Source: CAD feature listing. Evaluate the final solid. Frame: model axes, mm. Give positions to 0.01 mm unless a question says otherwise; leave off trailing zeros. Order: outer loops, then holes, each group sorted by start corner. A loop starts at its lowest first (then second) coordinate and runs counter-clockwise, first axis right, second up. Notation, with made-up numbers: M 87,49.25 L 146,49.25 A17 ccw 146,55.25 Z; hole C 43.5,-6.5 d7. An arc over 180 degrees is marked long. Answer as a JSON object with one key per item and string values. Group by question number.
1. Pin query (flat end, axial travel): P1, Ø1.6, axis at x = 46.99, y = 22.86, coming from the +Z side. Return the tip coordinate at first contact, or that it passes through.
2. Material intervals for L1, parallel to Y at x = 43.18, z = 0.45; L2, parallel to Y at x = 72.39, z = 1.2; L3, parallel to X at y = 10, z = 0.2, sorted ascending. Write a range as [from, to].
3. Pull-direction query (X, two-part tool) for faces 1 (the cylindrical face through (18.45, 2.98, 0.79)), 2 (the flat face through (5.08, 15, 1)), 3 (the cylindrical face through (94.47, 4.54, 0.79)), 4 (the flat face through (50, 0, 1)); classes: +X half, -X half, draft (parallel to the pull), parting line (faces both ways), or undercut.
4. Section query B-B (z = 0.3). Count the separate pieces of the cut face and the enclosed holes in it, plus the area to 3 significant figures.
5. Section query A-A (x = 72.39). Output: boundary loops of the cut face in (y, z).
Autodesk Inventor part; units mm, degrees
ref_plane "YZ Plane" through (0, 0, 0) normal (1, 0, 0) x (0, 1, 0)
ref_plane "XZ Plane" through (0, 0, 0) normal (0, 1, 0) x (-1, 0, 0)
ref_plane "XY Plane" through (0, 0, 0) normal (0, 0, 1) x (1, 0, 0)
sketch "Эскиз1" plane through (0, 0, 0) normal (0, 0, 1) x (1, 0, 0)
  line L0 (5.08, 0) -> (97.079, 0)
  line L1 (97.079, 0) -> (97.079, 30.47)
  line L2 (97.079, 30.47) -> (5.08, 30.47)
  line L3 (5.08, 30.47) -> (5.08, 0)
  circle A0 centre (46.99, 22.86) radius 0.6
  circle A1 centre (46.99, 20.32) radius 0.6
  circle A2 centre (46.99, 17.78) radius 0.6
  circle A3 centre (46.99, 15.24) radius 0.6
  circle A4 centre (46.99, 12.7) radius 0.6
  circle A5 centre (46.99, 10.16) radius 0.6
  circle A6 centre (46.99, 7.62) radius 0.6
  circle A7 centre (46.99, 5.08) radius 0.6
  circle A8 centre (54.61, 5.08) radius 0.6
  circle A9 centre (54.61, 7.62) radius 0.6
  circle A10 centre (54.61, 10.16) radius 0.6
  circle A11 centre (54.61, 12.7) radius 0.6
  circle A12 centre (54.61, 15.24) radius 0.6
  circle A13 centre (54.61, 17.78) radius 0.6
  circle A14 centre (54.61, 20.32) radius 0.6
  circle A15 centre (54.61, 22.86) radius 0.6
  circle A16 centre (8.89, 26.67) radius 1.905
  circle A17 centre (92.71, 3.81) radius 1.905
  circle A18 centre (16.51, 26.67) radius 1.905
  circle A19 centre (83.82, 3.81) radius 1.905
  circle A20 centre (33.02, 24.13) radius 0.51
  circle A21 centre (35.56, 24.13) radius 0.51
  circle A22 centre (38.1, 24.13) radius 0.51
  circle A23 centre (40.64, 24.13) radius 0.51
  circle A24 centre (10.1, 11.43) radius 1.15
  circle A25 centre (19.6, 19.83) radius 1.15
  circle A26 centre (19.6, 3.03) radius 1.15
  circle A27 centre (28, 11.43) radius 1.15
  circle A28 centre (20, 11.43) radius 1.15
  circle A29 centre (74.87, 19.05) radius 1.15
  circle A30 centre (84.37, 27.45) radius 1.15
  circle A31 centre (84.37, 10.65) radius 1.15
  circle A32 centre (92.77, 19.05) radius 1.15
  circle A33 centre (84.77, 19.05) radius 1.15
  circle A34 centre (24.13, 25.4) radius 1.5
  circle A35 centre (72.39, 3.81) radius 1.5
  circle A36 centre (43.18, 22.86) radius 0.5
  circle A37 centre (43.18, 12.7) radius 0.5
  circle A38 centre (38.1, 19.431) radius 0.5
  circle A39 centre (38.1, 13.335) radius 0.5
  circle A40 centre (38.1, 7.62) radius 0.5
  circle A41 centre (43.18, 7.62) radius 0.5
  circle A42 centre (62.23, 26.67) radius 0.5
  circle A43 centre (62.23, 7.62) radius 0.5
extrude "power_pcb.brdКонтур" add sketch "Эскиз1" along normal blind 1.6
properties part number "power_pcb.brdКонтур1"
Answer sheet:
{
 "1": {"P1": "z = 1.6"},
 "2": {"L1": "[0, 7.12], [8.12, 12.2], [13.2, 22.36], [23.36, 30.47]", "L2": "[0, 2.31], [5.31, 30.47]", "L3": "[5.08, 46.41], [47.57, 54.03], [55.19, 83.42], [85.32, 97.08]"},
 "3": {"face 1": "undercut", "face 2": "-X half", "face 3": "undercut", "face 4": "draft"},
 "4": {"separate pieces": "1", "enclosed holes": "44", "area": "2,670 mm^2"},
 "5": {"outline": "M 0,0 L 2.31,0 L 2.31,1.6 L 0,1.6 Z; M 5.31,0 L 30.47,0 L 30.47,1.6 L 5.31,1.6 Z"}
}
